Build history of the part. All positions in model axes, mm. A direction names the side the tool comes from. Round coordinates to 2 decimals unless told otherwise and drop trailing zeros. Write each loop counter-clockwise with the first axis right and the second up, starting at its lowest first coordinate (ties: lowest second). Pieces come first, ordered by that corner, then holes. Notation, with made-up numbers: M 6.25,70.25 L 14.25,70.25 A19 ccw 14.25,92.25 Z; hole C 4.25,82.25 d9. An arc over 180 degrees is marked long. Use a Markdown table: item, result.
from build123d import *

# Parameters (mm, degrees)
F1_DEPTH = 20
F2_R     = 2
F4_DEPTH = 2


with BuildPart() as f1:
    # F0 (on Front) → F1 (new body)
    with BuildSketch(Plane.XZ):
        Polygon((18, 18), (-18, 18), (-17, -18), (17, -18), align=None)
    extrude(amount=F1_DEPTH)

    # F2
    f2_edges = [f1.edges().sort_by_distance(p)[0] for p in [
        (-17, -10, -18),
        (-18, -10, 18),
        (18, -10, 18),
        (17, -10, -18),
        (17.5, -20, 0),
        (0, -20, -18),
        (-17.5, -20, 0),
        (0, -20, 18),
    ]]
    fillet(f2_edges, radius=F2_R)

    # F3 (on face) → F4 (cut)
    with BuildSketch(Plane.XZ.offset(20)):
        Polygon((-4, -12), (-4, 0), (-4, 12), (-12, 12), (-12, -12), align=None)
        Polygon((-5, 11), (-5, 0), (-5, -11), (-11, -11), (-11, 11), align=None, mode=Mode.SUBTRACT)
        with BuildLine():
            ThreePointArc((13, 0), (7, 6), (1, 0))
            ThreePointArc((1, 0), (7, -6), (13, 0))
        make_face()
        with BuildLine():
            ThreePointArc((12, 0), (7, -5), (2, 0))
            ThreePointArc((2, 0), (7, 5), (12, 0))
        make_face(mode=Mode.SUBTRACT)
    extrude(amount=-F4_DEPTH, mode=Mode.SUBTRACT)


solid = f1.part
Q1. Drop flat-ended pins along their axis: P1, Ø2, axis at y = -19.5, z = 5, coming from the +X side; P2, Ø2, axis at y = -19, z = -3.5, coming from the -X side; P3, Ø5, axis at y = -12, z = 2.5, coming from the -X side. Give the stop position or say it passes through.
Response values:
| item | result |
|---|---|
| P1 | stops at x = 17.58 |
| P2 | stops at x = -17.41 |
| P3 | stops at x = -17.64 |
Q2. Cut at A-A on y = -15.25. Give the cut face in (x, z).
Response values:
| item | result |
|---|---|
| outline | M -17.94,15.94 L -17.05,-16.06 A2 ccw -15.05,-18 L 15.05,-18 A2 ccw 17.05,-16.06 L 17.94,15.94 A2 ccw 15.94,18 L -15.94,18 A2 ccw Z |
Q3. Which spindle directions (+Z, -Z, +X, -X, +Y, -Y) get a long thin tool onto all of the face, cutting with end or side? Do faces 1 (the flat face through (-5, -19, 0)), 2 (the flat face through (7, -20, 0)). Say none if no direction does.
Response values:
| item | result |
|---|---|
| face 1 | -Y |
| face 2 | +Z, -Z, +X, -X, -Y |
Q4. Drill centre lines: L1, parallel to Z at x = 7, y = -18.45; L2, parallel to X at y = -19, z = 8; L3, parallel to Y at x = -11.5, z = 4.5. Where is each one in solid material? Low to high.
Response values:
| item | result |
|---|---|
| L1 | z = -17.95 to -6, -5 to 5, 6 to 17.95 |
| L2 | x = -17.45 to -12, -11 to -5, -4 to 17.45 |
| L3 | y = -18 to 0 |
Q5. Two-plate mould, pull along Z, no slides. Class faces 3 (the flat face through (0, 0, 0)), 4 (the flat face through (-8, -19, -12)), 5 (the cylindrical face through (16.43, -9.13, -17.45)): +Z half, -Z half, draft (parallel to the pull), parting line (faces both ways), or undercut.
Response values:
| item | result |
|---|---|
| face 3 | draft |
| face 4 | undercut |
| face 5 | -Z half |
